```python
from build123d import *

# Parameters (mm, degrees)
F1_DEPTH = 28.575
F2_R     = 12.7
F3_R     = 7.874
F4_DEPTH = 10.16


with BuildPart() as f1:
    # F0 (on Front) → F1 (new body, symmetric)
    with BuildSketch(Plane.XZ):
        with BuildLine():
            ThreePointArc((-19.05, 0), (0, 19.05), (19.05, 0))
            Line((19.05, 0), (59.69, 0))
            Line((59.69, 0), (59.69, -21.59))
            Line((59.69, -21.59), (69.85, -21.59))
            Line((69.85, -21.59), (69.85, 2.54))
            ThreePointArc((69.85, 2.54), (67.618154, 7.928154), (62.23, 10.16))
            Line((62.23, 10.16), (32.254, 10.16))
            ThreePointArc((32.254, 10.16), (28.378867, 11.218922), (25.580758, 14.101379))
            ThreePointArc((25.580758, 14.101379), (0, 29.21), (-25.580758, 14.101379))
            ThreePointArc((-25.580758, 14.101379), (-28.378867, 11.218922), (-32.254, 10.16))
            Line((-32.254, 10.16), (-62.23, 10.16))
            ThreePointArc((-62.23, 10.16), (-67.618154, 7.928154), (-69.85, 2.54))
            Line((-69.85, 2.54), (-69.85, -21.59))
            Line((-69.85, -21.59), (-59.69, -21.59))
            Line((-59.69, -21.59), (-59.69, 0))
            Line((-59.69, 0), (-19.05, 0))
        make_face()
    extrude(amount=F1_DEPTH, both=True)

    # F2
    f2_edges = [f1.edges().sort_by_distance(p)[0] for p in [
        (64.77, -28.575, -21.59),
        (-64.77, -28.575, -21.59),
        (64.77, 28.575, -21.59),
        (-64.77, 28.575, -21.59),
    ]]
    fillet(f2_edges, radius=F2_R)

    # F3 (on face) → F4 (cut)
    with BuildSketch(Plane.XY.offset(10.16)):
        with Locations((-44.45, 0)):
            Circle(F3_R)
        with Locations((44.45, 0)):
            Circle(F3_R)
    extrude(amount=-F4_DEPTH, mode=Mode.SUBTRACT)


solid = f1.part
```
Model file for the job. Use its own axes, mm. A direction names the side the tool comes from. Coordinates: 2 decimals unless noted, no trailing zeros. Loops run counter-clockwise (first coordinate to the right, second up) from the corner with the lowest first, then second, coordinate; pieces in that order, holes last. Notation, with made-up numbers: (-15.5, -13) - (-3.5, -13) arc R16 cw to (-3.5, 16) - close; hole circle Ø3 at (88, -23). An arc over 180 degrees is marked (long way). Answer as a JSON object with one key per item and string values. Group by question number.
(1) Cut at A-A (y = 0). Give the cut face in (x, z), then the cut area to 3 significant figures.
(2) Cut at D-D (y = 9.5). Give the cut face in (x, z).
(3) Cut at C-C (x = 44.45). Give the cut face in (y, z) (3 decimals).
(4) Two-plate mould, pull along X, no slides. Class faces 1 (the face through (64.841, -24.756, -17.968)), 2 (the face through (51.72, -3.02, 5.15)), 3 (the face through (-69.85, 0, -9)): released by +X, released by -X, zero draft, split by the parting line, or undercut.
(5) Flat gauge pins, fed straight in: pin 1 (15 mm diameter, centred on x = -47.5, y = -11, fed in from +Z); pin 2 (14 mm diameter, centred on x = 44.45, y = 0, fed in from -Z); pin 3 (8 mm diameter, centred on x = 40, y = 21, fed in from -Z); pin 4 (1.5 mm diameter, centred on y = 3.5, z = 16.5, fed in from -X). Where does each tip first touch, or does it go through?
(6) Tool access for faces 4 (the face through (-64.699, 24.756, -17.968)), 5 (the face through (-35, 0, 0)), 6 (the face through (54, 0, 10.16)): list every direction of +Z, -Z, +X, -X, +Y, -Y with a clear straight run to the whole face (end or side of a thin tool).
(7) Probe line 1 along Y through (x, z) = (44, 5) (3 decimals); line 2 along X through (y, z) = (19, -7); line 3 along X through (y, z) = (23, 1.5). List the from-to ranges inside material, lowest first.
(8) Cut at B-B (z = 8.5). Give the cut face in (x, y) (3 decimals), then the cut area to 3 significant figures.
Geometry says:
{
 "1": {"outline": "(-69.85, -21.59) - (-59.69, -21.59) - (-59.69, 0) - (-52.32, 0) - (-52.32, 10.16) - (-62.23, 10.16) arc R7.62 ccw to (-69.85, 2.54) - close; (-36.58, 0) - (-19.05, 0) arc R19.05 cw to (19.05, 0) - (36.58, 0) - (36.58, 10.16) - (32.25, 10.16) arc R7.62 cw to (25.58, 14.1) arc R29.21 ccw to (-25.58, 14.1) arc R7.62 cw to (-32.25, 10.16) - (-36.58, 10.16) - close; (52.32, 0) - (59.69, 0) - (59.69, -21.59) - (69.85, -21.59) - (69.85, 2.54) arc R7.62 ccw to (62.23, 10.16) - (52.32, 10.16) - close", "area": "1,710 mm^2"},
 "2": {"outline": "(-69.85, -21.59) - (-59.69, -21.59) - (-59.69, 0) - (-19.05, 0) arc R19.05 cw to (19.05, 0) - (59.69, 0) - (59.69, -21.59) - (69.85, -21.59) - (69.85, 2.54) arc R7.62 ccw to (62.23, 10.16) - (32.25, 10.16) arc R7.62 cw to (25.58, 14.1) arc R29.21 ccw to (-25.58, 14.1) arc R7.62 cw to (-32.25, 10.16) - (-62.23, 10.16) arc R7.62 ccw to (-69.85, 2.54) - close"},
 "3": {"outline": "(-28.575, 0) - (-7.874, 0) - (-7.874, 10.16) - (-28.575, 10.16) - close; (7.874, 0) - (28.575, 0) - (28.575, 10.16) - (7.874, 10.16) - close"},
 "4": {"face 1": "zero draft", "face 2": "undercut", "face 3": "released by -X"},
 "5": {"pin 1": "stops at z = 10.16", "pin 2": "passes through", "pin 3": "stops at z = 0", "pin 4": "stops at x = -24.6"},
 "6": {"face 4": "-Z, +X, -X, +Y", "face 5": "-Z, +Y, -Y", "face 6": "+Z, +X, +Y, -Y"},
 "7": {"line 1": "y = -28.575 to -7.861, 7.861 to 28.575", "line 2": "x = -69.85 to -59.69, 59.69 to 69.85", "line 3": "x = -69.85 to -18.99, 18.99 to 69.85"},
 "8": {"outline": "(-66.978, -28.575) - (-17.049, -28.575) - (-17.049, 28.575) - (-66.978, 28.575) - close; (17.049, -28.575) - (66.978, -28.575) - (66.978, 28.575) - (17.049, 28.575) - close; hole circle Ø15.748 at (-44.45, 0); hole circle Ø15.748 at (44.45, 0)", "area": "5,320 mm^2"}
}
